Study the drawing (mm; zero at the part's minimum x, y, z) and answer. Coordinates: 2 decimals unless noted, no trailing zeros. Loops run counter-clockwise (first coordinate to the right, second up) from the corner with the lowest first, then second, coordinate; pieces in that order, holes last. Notation, with made-up numbers: (-20.5, 49) - (-3.5, 49) arc R26 ccw to (-3.5, 71) - close; hole circle Ø7 at (28.25, 7). An arc over 180 degrees is marked (long way). Use CSV: the item, a comma, the result in double quotes.
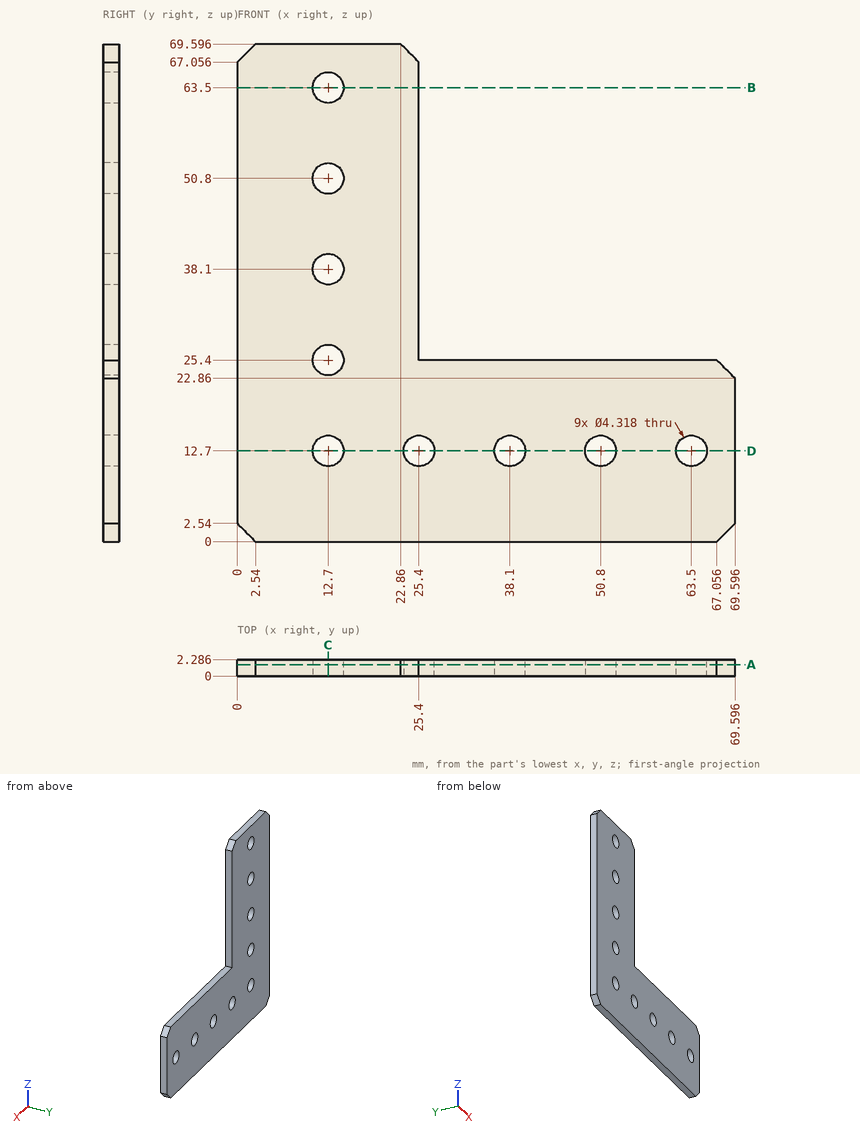
Q1. Find the intervals of material crossed by probe 1 along Z at (x, y) = (12.7, 1.25); probe 2 along X at (y, z) = (0.9, 63.5), in increasing order. Write a range as [from, to].
Reported:
probe 1,"z = [0, 10.54], [14.86, 23.24], [27.56, 35.94], [40.26, 48.64], [52.96, 61.34], [65.66, 69.6]"
probe 2,"x = [0, 10.54], [14.86, 25.4]"
Q2. The part is cut by section A-A on y = 1.6. Give the number of separate pieces and of enclosed holes in the cut face, and give its area (3 significant figures).
Reported:
separate pieces,"1"
enclosed holes,"9"
area,"2,740 mm²"
Q3. Given P1, Ø1.1, axis at x = 43, y = 1.5, coming from the +Z side, flat-ended and moving along its own axis, determine where the tip first touches the part or whether it passes through.
Reported:
P1,"stops at z = 25.4"
Q4. The part is cut by section D-D on z = 12.7. Determine the outline of the cut face in (x, y).
Reported:
outline,"(0, 0) - (10.54, 0) - (10.54, 2.29) - (0, 2.29) - close; (14.86, 0) - (23.24, 0) - (23.24, 2.29) - (14.86, 2.29) - close; (27.56, 0) - (35.94, 0) - (35.94, 2.29) - (27.56, 2.29) - close; (40.26, 0) - (48.64, 0) - (48.64, 2.29) - (40.26, 2.29) - close; (52.96, 0) - (61.34, 0) - (61.34, 2.29) - (52.96, 2.29) - close; (65.66, 0) - (69.6, 0) - (69.6, 2.29) - (65.66, 2.29) - close"
Q5. The part is cut by section B-B on z = 63.5. Determine the outline of the cut face in (x, y), and give its area (3 significant figures).
Reported:
outline,"(0, 0) - (10.54, 0) - (10.54, 2.29) - (0, 2.29) - close; (14.86, 0) - (25.4, 0) - (25.4, 2.29) - (14.86, 2.29) - close"
area,"48.2 mm²"
Q6. The part is cut by section C-C on x = 12.7. Determine the outline of the cut face in (y, z).
Reported:
outline,"(0, 0) - (2.29, 0) - (2.29, 10.54) - (0, 10.54) - close; (0, 14.86) - (2.29, 14.86) - (2.29, 23.24) - (0, 23.24) - close; (0, 27.56) - (2.29, 27.56) - (2.29, 35.94) - (0, 35.94) - close; (0, 40.26) - (2.29, 40.26) - (2.29, 48.64) - (0, 48.64) - close; (0, 52.96) - (2.29, 52.96) - (2.29, 61.34) - (0, 61.34) - close; (0, 65.66) - (2.29, 65.66) - (2.29, 69.6) - (0, 69.6) - close"
